Build history of the part. All positions in model axes, mm. A direction names the side the tool comes from. Give positions to 0.01 mm unless a question says otherwise; leave off trailing zeros. Answer as CSV lines item,"result".
from build123d import *

# Parameters (mm, degrees)
SKETCH070_R     = 1.6
PAD014_DEPTH    = 9
SKETCH071_R     = 1.5
POCKET033_DEPTH = 8
POCKET034_DEPTH = 9
SKETCH073_R     = 2
POCKET035_DEPTH = 7
SKETCH074_R     = 2
PAD015_DEPTH    = 5
SKETCH076_R     = 3.607909
SKETCH076_R_2   = 1.6
PAD016_DEPTH    = 9
SKETCH077_R     = 3
POCKET036_DEPTH = 5
CHAMFER_SIZE    = 0.5
FILLET001_R     = 0.5


with BuildPart() as part:
    # Sketch070 → Pad014 (new body)
    with BuildSketch(Plane.XY):
        with BuildLine():
            Line((-14.98648, 84.614769), (15.01352, 84.614769))
            Line((15.01352, 84.614769), (15.01352, 105.713058))
            Line((13.544477, 110.614769), (15.01352, 105.713058))
            ThreePointArc((13.544477, 110.614769), (0, 124.159246), (-13.544477, 110.614769))
            Line((-13.544477, 110.614769), (-14.98648, 105.713058))
            Line((-14.98648, 105.713058), (-14.98648, 84.614769))
        make_face()
        with Locations((11.3, 94.9)):
            Circle(SKETCH070_R, mode=Mode.SUBTRACT)
        with Locations((-11.1, 94.9)):
            Circle(SKETCH070_R, mode=Mode.SUBTRACT)
    extrude(amount=-PAD014_DEPTH)

    # Sketch071 → Pocket033 (cut)
    with BuildSketch(Plane.XY.offset(-1)):
        with Locations((0, 110.614769)):
            Circle(SKETCH071_R)
        with Locations((0, 114.114769)):
            Circle(SKETCH071_R)
        with Locations((0, 117.614769)):
            Circle(SKETCH071_R)
        with Locations((0, 121.114769)):
            Circle(SKETCH071_R)
        with Locations((0, 107.114769)):
            Circle(SKETCH071_R)
        with Locations((0, 103.614769)):
            Circle(SKETCH071_R)
        with Locations((0, 100.114769)):
            Circle(SKETCH071_R)
        with Locations((3.5, 110.614769)):
            Circle(SKETCH071_R)
        with Locations((7, 110.614769)):
            Circle(SKETCH071_R)
        with Locations((10.5, 110.614769)):
            Circle(SKETCH071_R)
        with Locations((-3.5, 110.614769)):
            Circle(SKETCH071_R)
        with Locations((-7, 110.614769)):
            Circle(SKETCH071_R)
        with Locations((-10.5, 110.614769)):
            Circle(SKETCH071_R)
        with Locations((3.5, 114.114769)):
            Circle(SKETCH071_R)
        with Locations((7, 114.114769)):
            Circle(SKETCH071_R)
        with Locations((-3.5, 114.114769)):
            Circle(SKETCH071_R)
        with Locations((-7, 114.114769)):
            Circle(SKETCH071_R)
        with Locations((3.5, 117.614769)):
            Circle(SKETCH071_R)
        with Locations((-3.5, 117.614769)):
            Circle(SKETCH071_R)
        with Locations((-3.5, 103.614769)):
            Circle(SKETCH071_R)
        with Locations((-3.5, 107.114769)):
            Circle(SKETCH071_R)
        with Locations((-7, 107.114769)):
            Circle(SKETCH071_R)
        with Locations((3.5, 103.614769)):
            Circle(SKETCH071_R)
        with Locations((3.5, 107.114769)):
            Circle(SKETCH071_R)
        with Locations((7, 107.114769)):
            Circle(SKETCH071_R)
    extrude(amount=-POCKET033_DEPTH, mode=Mode.SUBTRACT)

    # Sketch072 → Pocket034 (cut)
    with BuildSketch(Plane.XY.offset(-8)):
        with BuildLine():
            ThreePointArc((-13.403603, 92.74804), (-9.935518, 91.970581), (-7.947663, 94.916846))
            Line((-6.31942, 98.675576), (-7.947663, 94.916846))
            ThreePointArc((-6.31942, 98.675576), (-4.766235, 97.975053), (-3.137223, 97.47562))
            Line((-2.852251, 99.267758), (-3.137223, 97.47562))
            ThreePointArc((-7.50172, 101.636228), (-5.310705, 100.189492), (-2.852251, 99.267758))
            Line((-7.50172, 101.636228), (-8.942088, 100.500963))
            Line((-8.942088, 100.500963), (-10.804664, 98.038517))
            ThreePointArc((-10.804664, 98.038517), (-12.218753, 97.847186), (-13.403603, 97.05196))
            Line((-13.403603, 104.459993), (-13.403603, 97.05196))
            Line((-11.694871, 110.268376), (-13.403603, 104.459993))
            ThreePointArc((11.699959, 110.645764), (-0.188711, 122.313247), (-11.694871, 110.268376))
            Line((11.699959, 110.645764), (13.51352, 104.594511))
            Line((13.51352, 104.594511), (13.51352, 96.878203))
            Line((13.51352, 96.878203), (13.51352, 86.187889))
            Line((13.51352, 86.187889), (0, 86.187889))
            Line((-13.403603, 86.187889), (0, 86.187889))
            Line((-13.403603, 92.74804), (-13.403603, 86.187889))
        make_face()
    extrude(amount=POCKET034_DEPTH, mode=Mode.SUBTRACT)

    # Sketch073 → Pocket035 (cut)
    with BuildSketch(Plane.XY.offset(-8)):
        with Locations((5.937901, 89.530518)):
            Circle(SKETCH073_R)
        Polygon((-4.182843, 90.158684), (9.809951, 98.902352), (9.015072, 100.174424), (-4.977721, 91.430756), align=None)
    extrude(amount=-POCKET035_DEPTH, mode=Mode.SUBTRACT)

    # Sketch074 → Pad015 (join)
    with BuildSketch(Plane.XY.offset(-4)):
        with BuildLine():
            ThreePointArc((1.892431, 89.634359), (7.913794, 85.998881), (7.966013, 93.032428))
            ThreePointArc((7.695797, 94.813919), (7.403193, 93.858298), (7.966013, 93.032428))
            Line((7.695797, 94.813919), (11.764861, 99.227654))
            Line((11.764861, 99.227654), (13.51352, 98.900558))
            Line((13.51352, 98.900558), (13.51352, 104.594511))
            Line((13.51352, 104.594511), (13.091038, 106.004194))
            Line((10.100319, 102.55034), (13.091038, 106.004194))
            Line((10.100319, 102.55034), (9.489143, 103.770343))
            ThreePointArc((3.186255, 99.356981), (6.710877, 101.030713), (9.489143, 103.770343))
            ThreePointArc((3.186255, 99.356981), (2.297226, 98.856665), (1.734205, 98.005962))
            Line((1.734205, 98.005962), (1.165182, 96.436732))
            Line((1.165182, 96.436732), (-6.214738, 91.783745))
            Line((-6.214738, 91.783745), (-4.323315, 88.436639))
            Line((-4.323315, 88.436639), (0.140351, 90.734174))
            ThreePointArc((1.892431, 89.634359), (1.329754, 90.683475), (0.140351, 90.734174))
        make_face()
        with Locations((5.937901, 89.530518)):
            Circle(SKETCH074_R, mode=Mode.SUBTRACT)
        Polygon((-4.977721, 91.430756), (9.015072, 100.174424), (9.809951, 98.902352), (-4.182843, 90.158684), align=None, mode=Mode.SUBTRACT)
    extrude(amount=-PAD015_DEPTH)

    # Sketch076 → Pad016 (join)
    with BuildSketch(Plane.XY):
        with Locations((11.3, 94.9)):
            Circle(SKETCH076_R)
        with Locations((11.3, 94.9)):
            Circle(SKETCH076_R_2, mode=Mode.SUBTRACT)
    extrude(amount=-PAD016_DEPTH)

    # Sketch077 → Pocket036 (cut)
    with BuildSketch(Plane.XY.offset(-9)):
        with Locations((-11.1, 94.9)):
            Circle(SKETCH077_R)
        with Locations((11.3, 94.9)):
            Circle(SKETCH077_R)
    extrude(amount=POCKET036_DEPTH, mode=Mode.SUBTRACT)

    # Chamfer
    chamfer_edges = [part.edges().sort_by_distance(p)[0] for p in [
        (15.01352, 95.163913, -9),
        (-14.98648, 95.163913, -9),
    ]]
    chamfer(chamfer_edges, length=CHAMFER_SIZE)

    # Fillet001
    fillet001_edges = [part.edges().sort_by_distance(p)[0] for p in [
        (0, 124.159246, -9),
    ]]
    fillet(fillet001_edges, radius=FILLET001_R)


solid = part.part
Item 1: Probe line 1 along Y through (x, z) = (-8, -8.25); line 2 along Y through (x, z) = (-3.5, -1.25); line 3 along Y through (x, z) = (-10.5, -6.75). List the from-to ranges inside material, lowest first. Write a range as from..to.
Geometry says:
line 1,"y = 84.61..106, 108.23..109.5, 111.73..113, 115.23..121.54"
line 2,"y = 84.61..86.19, 97.57..99.45, 121.78..123.7"
line 3,"y = 84.61..86.19, 91.81..91.96, 97.84..98.44, 115.78..119.17"
Item 2: 3-axis set-ups, long thin cutter, end or side, ignore diameter. For faces 1 (the cylindrical face through (-0.2, 122.6, -5.9)), 2 (the flat face through (-9.86, 99.29, -4.06)), 3 (the flat face through (1.92, 95.74, -6.46)): which of +Z, -Z, +X, -X, +Y, -Y reach the whole face in a straight line?
Geometry says:
face 1,"-Z"
face 2,"+Z"
face 3,"+Z, -Z"
Item 3: Band-saw the part on A-A (z = -5.5). State how many separate pieces and enclosed holes the cut face has, and give its area (3 significant figures).
Geometry says:
separate pieces,"1"
enclosed holes,"8"
area,"348 mm2"
Item 4: Pull direction Y, two halves, no side cores. Call faces 4 (the cylindrical face through (-2.808, 109.284, -8.493)), 5 (the flat face through (13.514, 101, -2)): released by +Y, released by -Y, zero draft, split by the parting line, or undercut.
Geometry says:
face 4,"undercut"
face 5,"undercut"
Item 5: Drop flat-ended pins along their axis: pin 1 (3 mm diameter, centred on y = 120, z = -5.5, fed in from -X); pin 2 (2.5 mm diameter, centred on x = 3.5, y = 103.61, fed in from +Z); pin 3 (1 mm diameter, centred on x = 2.5, z = -8, fed in from +Y); pin 4 (1.5 mm diameter, centred on x = 5, z = -6.5, fed in from +Y). Give the stop position or say it passes through.
Geometry says:
pin 1,"stops at x = -11.01"
pin 2,"passes through"
pin 3,"stops at y = 124.01"
pin 4,"stops at y = 123.48"
